Autodesk Fusion 360 part; units mm, degrees
sketch "Sketch1" plane through (0, 0, 0) normal (0, 0, 1) x (1, 0, 0)
  circle A0 centre (0, 0) radius 13.7922 construction
  circle A1 centre (0, 0) radius 13.6525
  circle A2 centre (0, 0) radius 11.1525
  dimension "d1" = 27.5844
  dimension "d2" = 27.305
  dimension "d3" = 2.5
extrude "Extrude1" add sketch "Sketch1" against normal blind 38.1 contours A1 | A2
sketch "Sketch2" plane through (0, 0, 0) normal (1, 0, 0) x (0, 1, 0)
  line L0 (0, 0) -> (0, -39.2845) construction
  circle A0 centre (0, -25.4) radius 9.525
  line L1 (0, 0) -> (-28.4764, 0) construction
  circle A1 centre (0, -25.4) radius 12.7 construction
  line L2 (-13.6525, -38.1) -> (13.6525, -38.1) construction
  line L3 (-12.7, -38.1) -> (12.7, -38.1)
  line L4 (12.7, -38.1) -> (12.7, -17.78)
  line L5 (7.62, -12.7) -> (-7.62, -12.7)
  line L6 (-12.7, -17.78) -> (-12.7, -38.1)
  line L7 (-12.7, -38.1) -> (12.7, -12.7) construction
  line L8 (12.7, -38.1) -> (-12.7, -12.7) construction
  arc A2 (12.7, -17.78) -> (7.62, -12.7) centre (7.62, -17.78) ccw
  arc A3 (-7.62, -12.7) -> (-12.7, -17.78) centre (-7.62, -17.78) ccw
  point P0 (0, -25.4)
  dimension "d6" = 19.05
  dimension "d8" = 25.4
  dimension "d9" = 5.08
  dimension "d10" = 5.08
extrude "Extrude2" add sketch "Sketch2" against normal blind 19.05
extrude "Extrude3" cut sketch "Sketch2" against normal blind 34.8234 contours A0
extrude "Extrude4" cut sketch "Sketch1" against normal up to surface (37.38 mm away) contours A2
fillet "Fillet1" radius 0.508 1 edges at (-12.7286, -4.937, 0)
chamfer "Chamfer1" distance 1.27 angle 45 1 faces at (1.1599, 0.6789, -38.1)
chamfer "Chamfer2" distance 0.762 angle 45 1 edges at (-19.05, -8.8804, -28.8444)
Here's how the part is built. I have some questions about the finished solid (model axes, mm). A direction names the side the tool comes from. Coordinates: 2 decimals unless noted, no trailing zeros. Order: outer loops, then holes, each group sorted by start corner. A loop starts at its lowest first (then second) coordinate and runs counter-clockwise, first axis right, second up.
1) Imagine slicing it at B-B on x = -15.5. List the corners of the cut face in (y, z) for me (3 decimals).
2) I need wall thicknesses on line 1 (Y direction, x = 0, z = -18); line 2 (Y direction, x = -9, z = -25). Which ranges of each line are inside material? Lowest first, please.
3) Which directions (+Z, -Z, +X, -X, +Y, -Y) give clear straight access to the entire face, cutting with the end or side of a thin tool? Please do faces 4 (the face through (-13.492, -11.172, -14.149)), 5 (the face through (0, 0, -37.38)), 6 (the face through (-12, 12.7, -27)), 7 (the face through (-13.343, -9.516, -24.981)).
4) We'd pull the mould along X, two halves only. Please class faces 1 (the face through (10.637, 3.35, -18.428)), 2 (the face through (-11.81, -12.07, -37.46)), 3 (the face through (12.6, -0.35, -37.88)): +X half, -X half, draft (parallel to the pull), parting line (faces both ways), or undercut.
5) Imagine slicing it at D-D on x = 0. List the corners of the cut face in (y, z) for me, and give its area (3 significant figures).
6) Will these pins go through, and if not, where does the flat tip stop? pin 1 (11 mm diameter, centred on x = -10, z = -27, fed in from -Y); pin 2 (3 mm diameter, centred on x = 4, z = -22, fed in from +Y); pin 3 (8 mm diameter, centred on x = 5, z = -33, fed in from +Y).
Response values:
1. outline: (-12.7, -36.83) - (-11.43, -38.1) - (11.43, -38.1) - (12.7, -36.83) - (12.7, -17.78) arc R5.08 ccw to (7.62, -12.7) - (-7.62, -12.7) arc R5.08 ccw to (-12.7, -17.78) - close; hole circle Ø19.05 at (0, -25.4)
2. line 1: y = -13.65 to -11.15, 11.15 to 13.65
2. line 2: y = -12.7 to -9.52, 9.52 to 12.7
3. face 4: +Z, -X, -Y
3. face 5: +Z
3. face 6: +Z, -Z, -X, +Y
3. face 7: -X
4. face 1: undercut
4. face 2: draft
4. face 3: parting line
5. outline: (-13.65, -36.83) - (-12.38, -38.1) - (12.38, -38.1) - (13.65, -36.83) - (13.65, -0.51) arc R0.51 ccw to (13.14, 0) - (11.15, 0) - (11.15, -37.38) - (-11.15, -37.38) - (-11.15, 0) - (-13.14, 0) arc R0.51 ccw to (-13.65, -0.51) - close
5. area: 205 mm2
6. pin 1: stops at y = -12.89
6. pin 2: stops at y = 13.42
6. pin 3: stops at y = 13.62
